```python
from build123d import *

# Parameters (mm, degrees)
SKETCH001_AS_DRAWN_R                 = 6.35
SKETCH001_AS_DRAWN_R_2               = 1.27
EXTRUDE001_DEPTH                     = 76.2
EXTRUDE001_ONTO_SKETCH001_ROLL_ANGLE = 90
SKETCH_W                             = 88.9
SKETCH_H                             = 38.1
EXTRUDE_DEPTH                        = 419.1


with BuildPart() as extrude001:
    # Sketch001 as drawn → Extrude001 (new)
    with BuildSketch(Plane.XY):
        with Locations((44.45, 374.65)):
            Circle(SKETCH001_AS_DRAWN_R)
        with Locations((44.45, 38.1)):
            Circle(SKETCH001_AS_DRAWN_R)
        with Locations((31.75, 311.15)):
            Circle(SKETCH001_AS_DRAWN_R_2)
        with Locations((57.15, 311.15)):
            Circle(SKETCH001_AS_DRAWN_R_2)
        with Locations((31.75, 107.95)):
            Circle(SKETCH001_AS_DRAWN_R_2)
        with Locations((57.15, 107.95)):
            Circle(SKETCH001_AS_DRAWN_R_2)
    extrude(amount=-EXTRUDE001_DEPTH)


with BuildPart() as extrude001_1:
    # Extrude001 onto Sketch001 roll: moved
    add(extrude001.part.rotate(Axis((0, 0, 0), (1, 0, 0)), EXTRUDE001_ONTO_SKETCH001_ROLL_ANGLE))


with BuildPart() as extrude001_2:
    # Extrude001 onto Sketch001 placement: moved
    add(extrude001_1.part)


with BuildPart() as cut:
    # Sketch → Extrude (new body)
    with BuildSketch(Plane.XY):
        with Locations((44.45, 19.05)):
            Rectangle(SKETCH_W, SKETCH_H)
    extrude(amount=EXTRUDE_DEPTH)

    # Cut: cut Extrude001
    add(extrude001_2.part, mode=Mode.SUBTRACT)


solid = cut.part
```
Model file for the job. Use its own axes, mm. Round coordinates to 2 decimals unless told otherwise and drop trailing zeros. Loops run counter-clockwise (first coordinate to the right, second up) from the corner with the lowest first, then second, coordinate; pieces in that order, holes last. Notation, with made-up numbers: M -8,85.25 L 2,85.25 A17 cw 2,96.25 Z; hole C -19,6.5 d1. An arc over 180 degrees is marked long. Put each result on its own line as item: value. Start each with the question number.
Item 1: Drill centre lines: line 1 along Z through (x, y) = (44.45, 20.5); line 2 along Z through (x, y) = (31.75, 11); line 3 along X through (y, z) = (18, 311). Where is each one in solid material? Low to high.
Item 2: Cut at A-A (z = 38.1). List the corners of the cut face in (x, y), then the cut area to 3 significant figures.
Item 3: Mould opens along X. For faces 1 (the face through (44, 38.1, 207)), 2 (the face through (43.623, 18.783, 380.946)), 3 (the face through (0, 19, 207)) say: released by +X, released by -X, zero draft, split by the parting line, or undercut.
Answer block:
1. line 1: 0 to 31.75, 44.45 to 368.3, 381 to 419.1
1. line 2: 0 to 106.68, 109.22 to 309.88, 312.42 to 419.1
1. line 3: 0 to 30.49, 33.01 to 55.89, 58.41 to 88.9
2. outline: M 0,0 L 38.1,0 L 38.1,38.1 L 0,38.1 Z; M 50.8,0 L 88.9,0 L 88.9,38.1 L 50.8,38.1 Z
2. area: 2,900 mm2
3. face 1: zero draft
3. face 2: undercut
3. face 3: released by -X
